Verification items for this drawing (mm, ordinates from the low corner). A direction names the side the tool comes from. Round coordinates to 2 decimals unless told otherwise and drop trailing zeros. Order: outer loops, then holes, each group sorted by start corner. A loop starts at its lowest first (then second) coordinate and runs counter-clockwise, first axis right, second up. Notation, with made-up numbers: M 2.5,-32 L 40.5,-32 A18 ccw 40.5,-16 Z; hole C 74.25,-10.75 d10. An arc over 180 degrees is marked long. One line per item, written item: value. Start each with the question number.
(1) Cross-section at C-C, the plane y = 23. Enter the section's corners in (x, z).
(2) Depth check by flat-ended pin: pin 1 Ø1 at (x, y) = (9.5, 24.5) entering from +Z; pin 2 Ø1 at (y, z) = (23.5, 0.5) entering from +X; pin 3 Ø2 at (y, z) = (11, 1) entering from -X; pin 4 Ø2 at (x, y) = (16, 6) entering from -Z. Enter the tip coordinate at first touch or a pass-through.
(3) Thickness scan on L1, parallel to Z at x = 10, y = 19; L2, parallel to Y at x = 26.5, z = 5. Record the ranges inside material, lowest first.
(4) Cross-section at D-D, the plane x = 29. Enter the section's corners in (y, z).
(5) Cross-section at A-A, the plane x = 22.5. Enter the section's corners in (y, z).
(6) Access from +Z, -Z, +X, -X, +Y, -Y to the whole of each face (thin tool, end or side, straight path). Record for the marked faces 1 and 2.
(7) Cross-section at B-B, the plane z = 20.5. Enter the section's corners in (x, y).
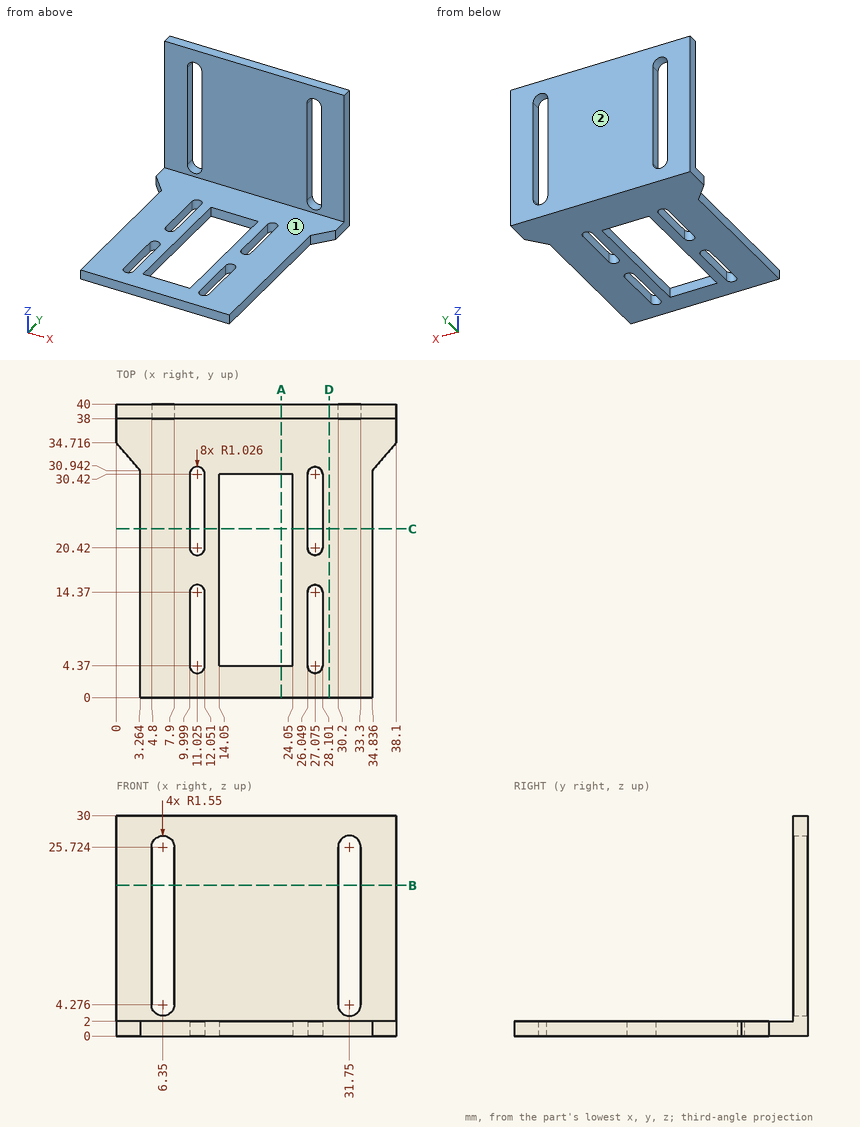
Values found:
1. outline: M 3.26,0 L 10,0 L 10,2 L 3.26,2 Z; M 12.05,0 L 14.05,0 L 14.05,2 L 12.05,2 Z; M 24.05,0 L 26.05,0 L 26.05,2 L 24.05,2 Z; M 28.1,0 L 34.84,0 L 34.84,2 L 28.1,2 Z
2. pin 1: z = 2
2. pin 2: x = 34.84
2. pin 3: x = 3.26
2. pin 4: through
3. L1: 0 to 2
3. L2: 38 to 40
4. outline: M 0,0 L 40,0 L 40,30 L 38,30 L 38,2 L 0,2 Z
5. outline: M 0,0 L 4.37,0 L 4.37,2 L 0,2 Z; M 30.42,0 L 40,0 L 40,30 L 38,30 L 38,2 L 30.42,2 Z
6. face 1: +Z, +X, -X, -Y
6. face 2: +Z, -Z, +X, -X, +Y
7. outline: M 0,38 L 4.8,38 L 4.8,40 L 0,40 Z; M 7.9,38 L 30.2,38 L 30.2,40 L 7.9,40 Z; M 33.3,38 L 38.1,38 L 38.1,40 L 33.3,40 Z
